from build123d import *

# Parameters (mm, degrees)
F0_W     = 57.15
F0_H     = 57.15
F1_DEPTH = 57.15
F2_T     = -5.08
F3_R     = 2.54
F4_DEPTH = 25.4
F5_R     = 3.81
F6_DEPTH = 25.4


with BuildPart() as f1:
    # F0 (on Top) → F1 (new body)
    with BuildSketch(Plane.XY):
        Rectangle(F0_W, F0_H)
    extrude(amount=F1_DEPTH)

    # F2
    f2_openings = [f1.faces().sort_by_distance(p)[0] for p in [
        (0, 0, 57.15),
        (28.575, 0, 28.575),
        (0, 28.575, 28.575),
        (-28.575, 0, 28.575),
    ]]
    offset(amount=F2_T, openings=f2_openings)

    # F3 (on face) → F4 (cut)
    with BuildSketch(Plane(origin=(0, -23.495, 0), x_dir=(-1, 0, 0), z_dir=(0, 1, 0))):
        with Locations((-21.082, 49.657)):
            Circle(F3_R)
        with Locations((21.082, 49.657)):
            Circle(F3_R)
        with Locations((-21.082, 12.573)):
            Circle(F3_R)
        with Locations((21.082, 12.573)):
            Circle(F3_R)
    extrude(amount=-F4_DEPTH, mode=Mode.SUBTRACT)

    # F5 (on face) → F6 (cut)
    with BuildSketch(Plane.XZ.offset(28.575)):
        with Locations((0, 28.575)):
            Circle(F5_R)
    extrude(amount=-F6_DEPTH, mode=Mode.SUBTRACT)


solid = f1.part
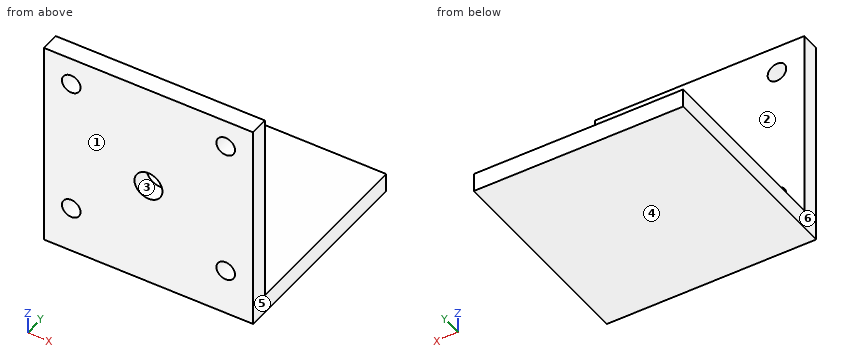
Geometry check sheet. Reference: the model listing, model coordinates, mm. Face numbers are marked on the shaded views. A direction names the side the tool comes from. Give positions to 0.01 mm unless a question says otherwise; leave off trailing zeros. Order: outer loops, then holes, each group sorted by start corner. A loop starts at its lowest first (then second) coordinate and runs counter-clockwise, first axis right, second up.
1. Scan lines: line 1 (Z direction, x = -9.5, y = -20.5); line 2 (Y direction, x = -16, z = 53.5) (3 decimals). Record each from-to range of solid material in increasing order.
Completed:
line 1: z = 0 to 5.08
line 2: y = -28.575 to -23.495
2. Sectioned sample at A-A (x = 0). Record the boundary of the cut face in (y, z) (3 decimals), then the cut area to 3 significant figures.
Completed:
outline: (-28.575, 0) - (28.575, 0) - (28.575, 5.08) - (-23.495, 5.08) - (-23.495, 24.765) - (-28.575, 24.765) - close; (-28.575, 32.385) - (-23.495, 32.385) - (-23.495, 57.15) - (-28.575, 57.15) - close
area: 516 mm2
3. Sectioned sample at D-D (z = 50.5). Record the boundary of the cut face in (x, y) (3 decimals), then the cut area to 3 significant figures.
Completed:
outline: (-28.575, -28.575) - (-23.478, -28.575) - (-23.478, -23.495) - (-28.575, -23.495) - close; (-18.686, -28.575) - (18.686, -28.575) - (18.686, -23.495) - (-18.686, -23.495) - close; (23.478, -28.575) - (28.575, -28.575) - (28.575, -23.495) - (23.478, -23.495) - close
area: 242 mm2
4. Access from +Z, -Z, +X, -X, +Y, -Y to the whole of each face (thin tool, end or side, straight path). Record for the marked faces 1 and 2.
Completed:
face 1: +Z, -Z, +X, -X, -Y
face 2: +Z, +X, -X, +Y
5. Depth check by flat-ended pin: pin 1 (8 mm diameter, centred on x = 4.5, y = -16.5, fed in from -Z); pin 2 (1 mm diameter, centred on x = 15, y = 21.5, fed in from +Z); pin 3 (6 mm diameter, centred on x = 21.082, z = 49.657, fed in from +Y) (3 decimals). Enter the tip coordinate at first touch or a pass-through.
Completed:
pin 1: stops at z = 0
pin 2: stops at z = 5.08
pin 3: stops at y = -23.495
6. Sectioned sample at B-B (z = 26.5). Record the boundary of the cut face in (x, y) (3 decimals), then the cut area to 3 significant figures.
Completed:
outline: (-28.575, -28.575) - (-3.195, -28.575) - (-3.195, -23.495) - (-28.575, -23.495) - close; (3.195, -28.575) - (28.575, -28.575) - (28.575, -23.495) - (3.195, -23.495) - close
area: 258 mm2
7. Sectioned sample at C-C (x = 21). Record the boundary of the cut face in (y, z) (3 decimals).
Completed:
outline: (-28.575, 0) - (28.575, 0) - (28.575, 5.08) - (-23.495, 5.08) - (-23.495, 10.034) - (-28.575, 10.034) - close; (-28.575, 15.112) - (-23.495, 15.112) - (-23.495, 47.118) - (-28.575, 47.118) - close; (-28.575, 52.196) - (-23.495, 52.196) - (-23.495, 57.15) - (-28.575, 57.15) - close
8. Draft check along X on the marked faces 3, 4, 5 and 6. Enter one of: pulls with the +X half, pulls with the -X half, needs draft (parallel to the pull), parting line crosses it, or undercut.
Completed:
face 3: undercut
face 4: needs draft
face 5: pulls with the +X half
face 6: pulls with the -X half
